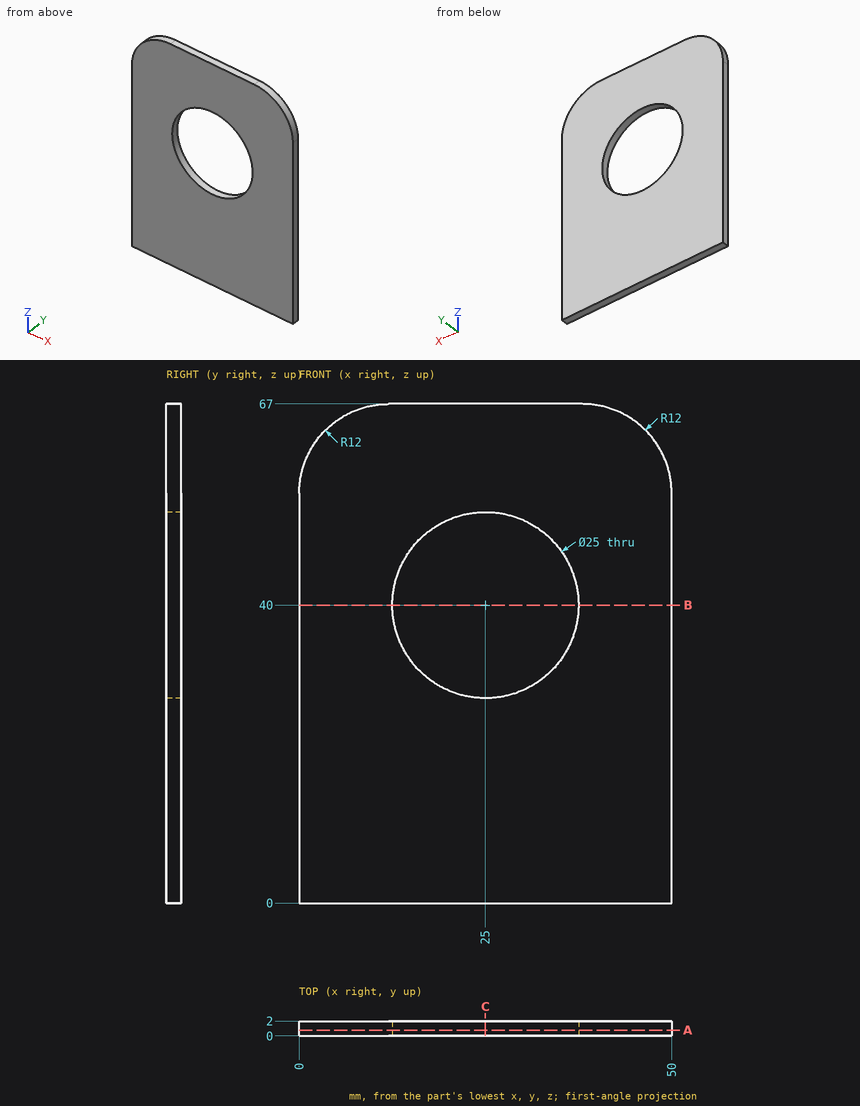
Geometry: see drawing. Coordinates: mm, zero at the bounding-box minimum. Round coordinates to 2 decimals unless told otherwise and drop trailing zeros. Loops run counter-clockwise (first coordinate to the right, second up) from the corner with the lowest first, then second, coordinate; pieces in that order, holes last. Notation, with made-up numbers: M 83,33.5 L 134,33.5 A19 ccw 134,68.5 Z; hole C -25.75,41 d8. An arc over 180 degrees is marked long. Use a Markdown table: item, result. Add a question column.
1. Cut plane A-A, the plane y = 0.8. Output: boundary loops of the cut face in (x, z).
2. Cut plane B-B, the plane z = 40. Output: boundary loops of the cut face in (x, y).
3. Cut plane C-C, the plane x = 25. Output: boundary loops of the cut face in (y, z).
4. Ray query, line 1 along Z through (x, y) = (25, 1.35); line 2 along Z through (x, y) = (36, 1.7); line 3 along X through (y, z) = (1.85, 48.5). Return the intervals inside material, ascending. Write a range as [from, to].
Solution:
| question | item | result |
|---|---|---|
| 1 | outline | M 0,0 L 50,0 L 50,55 A12 ccw 38,67 L 12,67 A12 ccw 0,55 Z; hole C 25,40 d25 |
| 2 | outline | M 0,0 L 12.5,0 L 12.5,2 L 0,2 Z; M 37.5,0 L 50,0 L 50,2 L 37.5,2 Z |
| 3 | outline | M 0,0 L 2,0 L 2,27.5 L 0,27.5 Z; M 0,52.5 L 2,52.5 L 2,67 L 0,67 Z |
| 4 | line 1 | z = [0, 27.5], [52.5, 67] |
| 4 | line 2 | z = [0, 34.06], [45.94, 67] |
| 4 | line 3 | x = [0, 15.83], [34.17, 50] |
